Can you work these out from the model? Positions are in its coordinate system, mm. Round coordinates to 2 decimals unless told otherwise and drop trailing zeros. Order: outer loops, then holes, each group sorted by start corner. A loop starts at its lowest first (then second) coordinate and runs counter-clockwise, first axis right, second up. Notation, with made-up numbers: (4.25, 8) -> (61.25, 8) arc R18 ccw to (61.25, 32) -> close; hole circle Ø1 at (40.25, 51.5). An arc over 180 degrees is marked (long way). Use a Markdown table: item, result. Add a question column.
Q1. If we section it at B-B on y = 7.25: List the corners of the cut face in (x, z) for me.
Q2. I need wall thicknesses on line 1 along Y through (x, z) = (56, 0.9); line 2 along X through (y, z) = (4.5, 2); line 3 along X through (y, z) = (5.5, 1.2). Which ranges of each line are inside material? Lowest first, please. Write a range as [from, to].
Q3. If we section it at A-A on z = 2.15: List the corners of the cut face in (x, y) for me.
Q4. I'm going to push a flat-ended pin straight in: pin 1 Ø1.5 at (y, z) = (1.5, 2.5) entering from +X. Where does the tip first touch, or does it pass through?
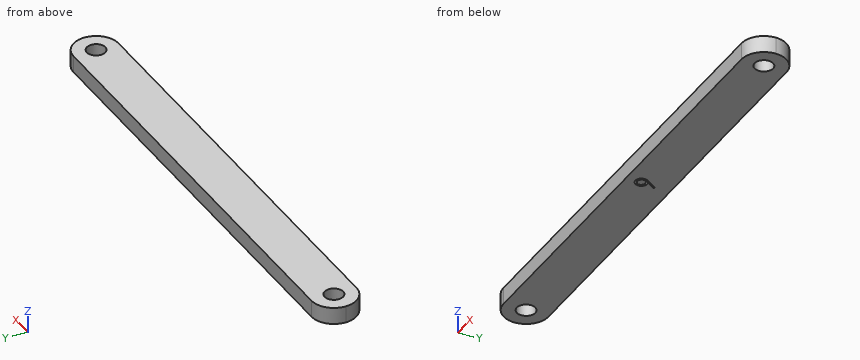
```python
from build123d import *

# Parameters (mm, degrees)
SKETCH_1_R          = 1.3
SKETCH_1_R_2        = 1.65
EXTRUDE_1_DEPTH     = 3
SKETCH_2_R          = 1.65
CUT_EXTRUDE_1_DEPTH = 61.466769186
CUT_EXTRUDE_2_DEPTH = 1


with BuildPart() as part:
    # 草图1 → 凸台-拉伸1 (new body)
    with BuildSketch(Plane(origin=(0, 0, 0), x_dir=(-1, 0, 0), z_dir=(0, 0, -1))):
        with BuildLine():
            Line((-55.860221974, 0), (24.13832066, 0))
            ThreePointArc((24.13832066, 0), (26.966394209, 1.171219344), (28.138320535, 3.999))
            ThreePointArc((28.138320535, 3.999), (26.96674766, 6.827427125), (24.138320535, 7.999))
            Line((24.138320535, 7.999), (-55.860222099, 7.999))
            ThreePointArc((-55.860222099, 7.999), (-58.688295648, 6.827780656), (-59.860221974, 4))
            ThreePointArc((-59.860221974, 4), (-58.688649099, 1.171572875), (-55.860221974, 0))
        make_face()
        with Locations((24.138809001, 3.998511534)):
            Circle(SKETCH_1_R, mode=Mode.SUBTRACT)
        with Locations((-55.859733508, 3.999511534)):
            Circle(SKETCH_1_R_2, mode=Mode.SUBTRACT)
    extrude(amount=-EXTRUDE_1_DEPTH)

    # 草图2 → 切除-拉伸1 (cut, through all)
    with BuildSketch(Plane.XY.offset(3)):
        with Locations((-24.138809001, 3.998511534)):
            Circle(SKETCH_2_R)
    extrude(amount=-CUT_EXTRUDE_1_DEPTH, mode=Mode.SUBTRACT)

    # 草图3 → 切除-拉伸2 (cut)
    with BuildSketch(Plane(origin=(0, 0, 0), x_dir=(-1, 0, 0), z_dir=(0, 0, -1))):
        with BuildLine():
            Line((-16.710668713, 5.336154662), (-16.468781693, 5.146150656))
            Line((-16.468781693, 5.146150656), (-17.393561341, 3.731987996))
            add(Edge.make_bspline(
                [(-17.393561341, 3.731987996), (-17.331991064, 3.741801856), (-17.211891277, 3.760944901), (-17.090325379, 3.764102847), (-17.031081373, 3.765641842)],
                knots=[0, 0, 0, 0, 1.025318673, 2, 2, 2, 2], degree=3))
            add(Edge.make_bspline(
                [(-17.031081373, 3.765641842), (-16.995508877, 3.76468573), (-16.925485476, 3.762803653), (-16.822678674, 3.748319802), (-16.723889738, 3.72549469), (-16.629528126, 3.692222434), (-16.539255144, 3.64972008), (-16.452552748, 3.59878121), (-16.371050738, 3.536775529), (-16.293699558, 3.467510573), (-16.223472461, 3.390793589), (-16.161296405, 3.309392252), (-16.109069614, 3.223391371), (-16.066695692, 3.132834505), (-16.033790813, 3.037861246), (-16.009803168, 2.938593106), (-15.995623576, 2.834961635), (-15.993698085, 2.76448346), (-15.992719995, 2.728682707)],
                knots=[0, 0, 0, 0, 1.04369286, 2.054478336, 3.041073146, 4.015093852, 4.984733326, 5.965804835, 6.960378782, 7.985147595, 9.009457201, 10.008161701, 10.986880575, 11.956520048, 12.937015923, 13.931873656, 14.949455224, 16, 16, 16, 16], degree=3))
            add(Edge.make_bspline(
                [(-15.992719995, 2.728682707), (-15.9941431, 2.679703003), (-15.996943433, 2.583322537), (-16.024847229, 2.442945831), (-16.068206874, 2.309213315), (-16.130184402, 2.184260144), (-16.207166785, 2.068257574), (-16.301044378, 1.965472109), (-16.408487866, 1.873802072), (-16.529974665, 1.797145453), (-16.660717629, 1.734542402), (-16.798069626, 1.689577159), (-16.940696772, 1.66189369), (-17.03750138, 1.658423087), (-17.086469995, 1.656667483)],
                knots=[0, 0, 0, 0, 1.031375318, 2.029502543, 3.004789286, 3.987476834, 4.960371455, 5.9300674, 6.912260825, 7.929083631, 8.949397511, 9.960523116, 10.96833055, 12, 12, 12, 12], degree=3))
            add(Edge.make_bspline(
                [(-17.086469995, 1.656667483), (-17.133566695, 1.658195689), (-17.226857013, 1.661222797), (-17.364089808, 1.688188735), (-17.495952825, 1.731895837), (-17.621522206, 1.792110116), (-17.737842819, 1.868167999), (-17.841908455, 1.959730278), (-17.93320023, 2.064839743), (-18.009174851, 2.18348009), (-18.069433583, 2.310970048), (-18.114623508, 2.443907204), (-18.141019751, 2.581807186), (-18.144708308, 2.675288325), (-18.146566149, 2.722372611)],
                knots=[0, 0, 0, 0, 1.012016664, 2.004627821, 2.994792927, 3.992885782, 4.990978636, 5.973936114, 6.964471063, 7.975201453, 8.993600317, 9.990122807, 10.98767138, 12, 12, 12, 12], degree=3))
            add(Edge.make_bspline(
                [(-18.146566149, 2.722372611), (-18.145384704, 2.758417194), (-18.142972419, 2.832013346), (-18.126129028, 2.943477374), (-18.099064233, 3.057528456), (-18.068753987, 3.15428265), (-18.036728377, 3.233544172), (-18.010075837, 3.297447662), (-17.976901841, 3.363208735), (-17.94152846, 3.433082371), (-17.900771591, 3.505267804), (-17.856455942, 3.580971474), (-17.807356291, 3.658989401), (-17.772936128, 3.711933596), (-17.755340187, 3.738999214)],
                knots=[0, 0, 0, 0, 1.173818275, 2.396712641, 3.66331629, 4.989737886, 5.693666774, 6.447286557, 7.243889047, 8.091586357, 8.998013824, 9.943181721, 10.948533338, 12, 12, 12, 12], degree=3))
            Line((-17.755340187, 3.738999214), (-16.710668713, 5.336154662))
        make_face()
        with BuildLine():
            add(Edge.make_bspline(
                [(-17.096986822, 3.406667483), (-17.123649066, 3.405889439), (-17.175728176, 3.404369694), (-17.252135591, 3.395544442), (-17.324448842, 3.378925376), (-17.393625976, 3.357759044), (-17.458373679, 3.328655985), (-17.519162518, 3.293304186), (-17.57622757, 3.251683008), (-17.628971122, 3.204382096), (-17.676790785, 3.152594064), (-17.717971916, 3.097124541), (-17.753494316, 3.039310338), (-17.782376135, 2.978668396), (-17.804866211, 2.915221896), (-17.821134462, 2.849262647), (-17.830188213, 2.780348341), (-17.831694444, 2.733615838), (-17.832463584, 2.709752419)],
                knots=[0, 0, 0, 0, 1.129588631, 2.206414736, 3.251139165, 4.268635594, 5.265702196, 6.250456724, 7.242448911, 8.251968645, 9.246821453, 10.222880186, 11.173611482, 12.116736599, 13.062300278, 14.020270554, 14.989073742, 16, 16, 16, 16], degree=3))
            add(Edge.make_bspline(
                [(-17.832463584, 2.709752419), (-17.831837223, 2.686102439), (-17.830609021, 2.639728349), (-17.819456701, 2.57138917), (-17.802421619, 2.505624261), (-17.777081223, 2.442772662), (-17.746854335, 2.381876344), (-17.706949011, 2.325141059), (-17.662732225, 2.269120989), (-17.609878292, 2.218119517), (-17.553154929, 2.170662893), (-17.492553726, 2.12918264), (-17.429393766, 2.093696466), (-17.362822344, 2.065885369), (-17.29378396, 2.043061082), (-17.221703406, 2.026999603), (-17.146530551, 2.017919077), (-17.095608613, 2.016410883), (-17.069643072, 2.015641842)],
                knots=[0, 0, 0, 0, 0.989467248, 1.94019797, 2.891935182, 3.827694429, 4.772920941, 5.730924762, 6.725747692, 7.756678648, 8.79901574, 9.819492441, 10.826891316, 11.826466727, 12.835195252, 13.867842842, 14.912794438, 16, 16, 16, 16], degree=3))
            add(Edge.make_bspline(
                [(-17.069643072, 2.015641842), (-17.043677573, 2.016410943), (-16.992755718, 2.017919255), (-16.917582258, 2.026998924), (-16.84550394, 2.043063572), (-16.776457431, 2.065876342), (-16.709916, 2.093729952), (-16.646811278, 2.128961871), (-16.586783185, 2.170917989), (-16.530022585, 2.218038417), (-16.477388647, 2.269411269), (-16.432111368, 2.324640992), (-16.393428135, 2.382334887), (-16.361993948, 2.442532777), (-16.336932657, 2.505662265), (-16.319811189, 2.571378989), (-16.3086819, 2.639731015), (-16.307450534, 2.686103339), (-16.306822559, 2.709752419)],
                knots=[0, 0, 0, 0, 1.087397944, 2.132534446, 3.165364764, 4.174271784, 5.174024072, 6.181601208, 7.194203697, 8.236725232, 9.267838612, 10.269026844, 11.221737037, 12.171628256, 13.107553087, 14.05945871, 15.010357665, 16, 16, 16, 16], degree=3))
            add(Edge.make_bspline(
                [(-16.306822559, 2.709752419), (-16.307372852, 2.73364697), (-16.308452898, 2.780544202), (-16.320668847, 2.84923182), (-16.33761122, 2.915557027), (-16.363194251, 2.979102976), (-16.396430796, 3.039618903), (-16.436914203, 3.097410504), (-16.483746773, 3.152920851), (-16.537844313, 3.20448366), (-16.596734547, 3.251630737), (-16.659350132, 3.293250294), (-16.724858106, 3.328375271), (-16.793192048, 3.357682373), (-16.865134931, 3.378831847), (-16.93952527, 3.39548509), (-17.017314513, 3.404347108), (-17.070091121, 3.405884173), (-17.096986822, 3.406667483)],
                knots=[0, 0, 0, 0, 0.978206639, 1.919901502, 2.851605144, 3.780102724, 4.718870031, 5.675451981, 6.667674623, 7.690630536, 8.733308323, 9.756129687, 10.767539656, 11.776269907, 12.797430371, 13.836405707, 14.897401972, 16, 16, 16, 16], degree=3))
        make_face(mode=Mode.SUBTRACT)
    extrude(amount=-CUT_EXTRUDE_2_DEPTH, mode=Mode.SUBTRACT)


solid = part.part
```
Answer below:
| question | item | result |
|---|---|---|
| 1 | outline | (-26.47, 0) -> (58.19, 0) -> (58.19, 3) -> (-26.47, 3) -> close |
| 2 | line 1 | [0, 2.36], [5.64, 8] |
| 2 | line 2 | [-28.11, -25.71], [-22.57, 54.29], [57.43, 59.83] |
| 2 | line 3 | [-27.85, -24.82], [-23.45, 55.17], [56.55, 59.57] |
| 3 | outline | (-28.14, 4) arc R4 ccw to (-24.14, 0) -> (55.86, 0) arc R4 ccw to (59.86, 4) arc R4 ccw to (55.86, 8) -> (-24.14, 8) arc R4 ccw to start; hole circle Ø3.3 at (-24.14, 4); hole circle Ø3.3 at (55.86, 4) |
| 4 | pin 1 | x = 59.46 |
